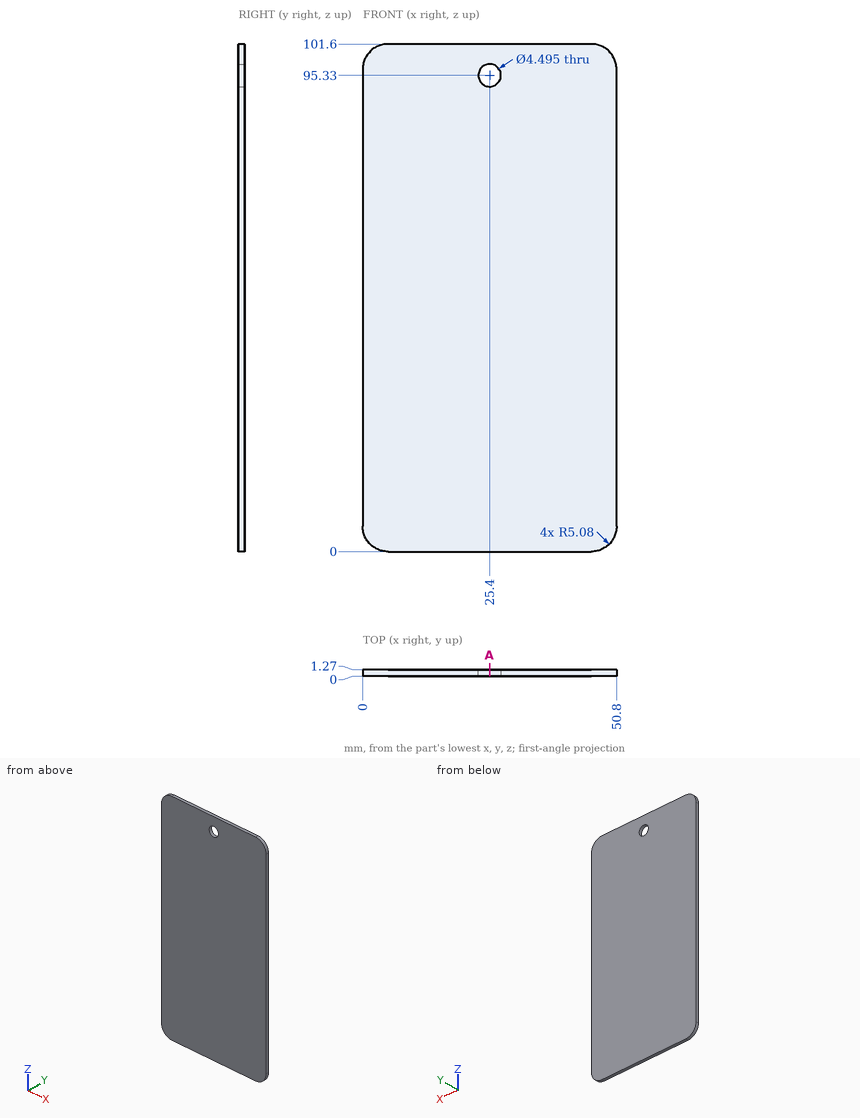
Can you work these out from the drawing? Everything is in mm from the part's minimum corner. Coordinates: 2 decimals unless noted, no trailing zeros. Loops run counter-clockwise (first coordinate to the right, second up) from the corner with the lowest first, then second, coordinate; pieces in that order, holes last. Notation, with made-up numbers: M -27,61 L 9,61 A6 cw 9,70 Z; hole C 36,-21.75 d4. An arc over 180 degrees is marked long. Put each result on its own line as item: value. Start each with the question number.
(1) I need wall thicknesses on line 1 (Z direction, x = 25.4, y = 0.9); line 2 (X direction, y = 0.45, z = 94.5); line 3 (Z direction, x = 4, y = 1.15) (1 decimal). Which ranges of each line are inside material? Lowest first, please. Write a range as from..to.
(2) Will this pin go through, and if not, where does the flat tip stop? P1, Ø4, axis at x = 8.5, z = 35, coming from the -Y side.
(3) Suppose I cut it at A-A on x = 25.4. Please give me the cut outline in (y, z).
Solutions:
1. line 1: z = 0..93.08, 97.58..101.6
1. line 2: x = 0..23.31, 27.49..50.8
1. line 3: z = 0.1..101.5
2. P1: stops at y = 0
3. outline: M 0,0 L 1.27,0 L 1.27,93.08 L 0,93.08 Z; M 0,97.58 L 1.27,97.58 L 1.27,101.6 L 0,101.6 Z
